The model under review builds one solid part; all positions refer to its coordinate system, in mm. A direction names the side the tool comes from. Round coordinates to 2 decimals unless told otherwise and drop trailing zeros. Write each loop counter-clockwise with the first axis right and the second up, starting at its lowest first coordinate (ties: lowest second). Pieces come first, ordered by that corner, then holes. Notation, with made-up numbers: (4, 31.5) - (60, 31.5) arc R23 ccw to (60, 70.5) - close; hole circle Ø9 at (-8.75, 53.25). An arc over 180 degrees is marked (long way). Use one line per item in the form item = value.
from build123d import *

# Parameters (mm, degrees)
SKETCH2_R           = 7.5
BOSS_EXTRUDE1_DEPTH = 10
BOSS_EXTRUDE3_START = 3
SKETCH4_R           = 30
SKETCH4_R_2         = 4.25
BOSS_EXTRUDE3_DEPTH = 3
BOSS_EXTRUDE4_START = 3
SKETCH5_R           = 30
BOSS_EXTRUDE4_DEPTH = 3
BOSS_EXTRUDE5_START = 10
SKETCH6_R           = 7.5
BOSS_EXTRUDE5_DEPTH = 10


with BuildPart() as part:
    # Sketch2 → Boss-Extrude1 (new body)
    with BuildSketch(Plane.XY):
        Circle(SKETCH2_R)
        with BuildLine():
            ThreePointArc((-1.565247584, 2.2), (0, -2.7), (1.565247584, 2.2))
            Line((1.565247584, 2.2), (-1.565247584, 2.2))
        make_face(mode=Mode.SUBTRACT)
    extrude(amount=-BOSS_EXTRUDE1_DEPTH)

    # Sketch4 → Boss-Extrude3 (add)
    with BuildSketch(Plane.XY.offset(BOSS_EXTRUDE3_START)):
        Circle(SKETCH4_R)
        with Locations((-16.970562748, -16.970562748)):
            Circle(SKETCH4_R_2, mode=Mode.SUBTRACT)
        with Locations((-24, 0)):
            Circle(SKETCH4_R_2, mode=Mode.SUBTRACT)
        with Locations((0, -24)):
            Circle(SKETCH4_R_2, mode=Mode.SUBTRACT)
        with Locations((16.970562748, -16.970562748)):
            Circle(SKETCH4_R_2, mode=Mode.SUBTRACT)
        with Locations((-16.970562748, 16.970562748)):
            Circle(SKETCH4_R_2, mode=Mode.SUBTRACT)
        with Locations((24, 0)):
            Circle(SKETCH4_R_2, mode=Mode.SUBTRACT)
        with Locations((0, 24)):
            Circle(SKETCH4_R_2, mode=Mode.SUBTRACT)
        with Locations((16.970562748, 16.970562748)):
            Circle(SKETCH4_R_2, mode=Mode.SUBTRACT)
        with BuildLine():
            ThreePointArc((1.565247584, 2.2), (0, -2.7), (-1.565247584, 2.2))
            Line((-1.565247584, 2.2), (1.565247584, 2.2))
        make_face(mode=Mode.SUBTRACT)
    extrude(amount=-BOSS_EXTRUDE3_DEPTH)

    # Sketch5 → Boss-Extrude4 (add)
    with BuildSketch(Plane.XY.offset(3).offset(BOSS_EXTRUDE4_START)):
        Circle(SKETCH5_R)
    extrude(amount=-BOSS_EXTRUDE4_DEPTH)

    # Sketch6 → Boss-Extrude5 (add)
    with BuildSketch(Plane.XY.offset(6).offset(BOSS_EXTRUDE5_START)):
        Circle(SKETCH6_R)
        with BuildLine():
            Line((1.565247584, 2.2), (-1.565247584, 2.2))
            ThreePointArc((-1.565247584, 2.2), (0, -2.7), (1.565247584, 2.2))
        make_face(mode=Mode.SUBTRACT)
    extrude(amount=-BOSS_EXTRUDE5_DEPTH)


solid = part.part
(1) Add section D-D on y = 0. Write out the cut boundary in (x, z).
Geometry results:
outline = (-30, 0) - (-28.25, 0) - (-28.25, 3) - (-19.75, 3) - (-19.75, 0) - (-7.5, 0) - (-7.5, -10) - (-2.7, -10) - (-2.7, 3) - (2.7, 3) - (2.7, -10) - (7.5, -10) - (7.5, 0) - (19.75, 0) - (19.75, 3) - (28.25, 3) - (28.25, 0) - (30, 0) - (30, 6) - (7.5, 6) - (7.5, 16) - (2.7, 16) - (2.7, 6) - (-2.7, 6) - (-2.7, 16) - (-7.5, 16) - (-7.5, 6) - (-30, 6) - close
(2) Insertion check: P1, Ø1.6, axis at x = 0, z = 12, coming from the -Y side; P2, Ø8, axis at y = -6, z = 1.5, coming from the +X side; P3, Ø3, axis at x = 0, y = 0, coming from the +Z side. Each pin has a flat end and moves straight along its axis. Give the tip position at first contact, or say it passes through.
Geometry results:
P1 = -7.5
P2 = 29.93
P3 = 6
(3) Add section C-C on z = -4.25. Write out the cut boundary in (x, y), then the cut area to 3 significant figures.
Geometry results:
outline = circle Ø15 at (0, 0); hole (-1.57, 2.2) arc R2.7 ccw (long way) to (1.57, 2.2) - close
area = 155 mm2
(4) The part is to be moulded in two halves that separate along Y. For faces 1 (the flat face through (17, -17, 3)), 2 (the cylindrical face through (-29.97, 1.32, 3.04)), 3 (the flat face through (-24, 0, 3)), 4 (the flat face through (6, -6, 0)), say which applies: +Y half, -Y half, draft (parallel to the pull), parting line (faces both ways), or undercut.
Geometry results:
face_1 = undercut
face_2 = parting line
face_3 = undercut
face_4 = draft
(5) Machinability: for faces 5 (the cylindrical face through (-0.92, -28.15, 1.52)), 6 (the flat face through (0, 0, 6)), which of the approach directions +Z, -Z, +X, -X, +Y, -Y give a long, thin tool a straight path to every point of the face, cutting with its end or side? Answer none if there is none.
Geometry results:
face_5 = -Z
face_6 = +Z
(6) To check wall thickness, follow L1, parallel to Y at x = 0, z = 0.9; L2, parallel to Y at x = 0, z = -6.5; L3, parallel to Y at x = 14.5, z = 1.25. State the ranges of each line that lie inside material, in increasing order.
Geometry results:
L1 = -30 to -28.25, -19.75 to -2.7, 2.2 to 19.75, 28.25 to 30
L2 = -7.5 to -2.7, 2.2 to 7.5
L3 = -26.26 to -20.43, -13.51 to 13.51, 20.43 to 26.26
(7) Add section A-A on y = -24. Write out the cut boundary in (x, z), then the cut area to 4 significant figures.
Geometry results:
outline = (-18, 0) - (-4.25, 0) - (-4.25, 3) - (4.25, 3) - (4.25, 0) - (18, 0) - (18, 6) - (-18, 6) - close
area = 190.5 mm2
